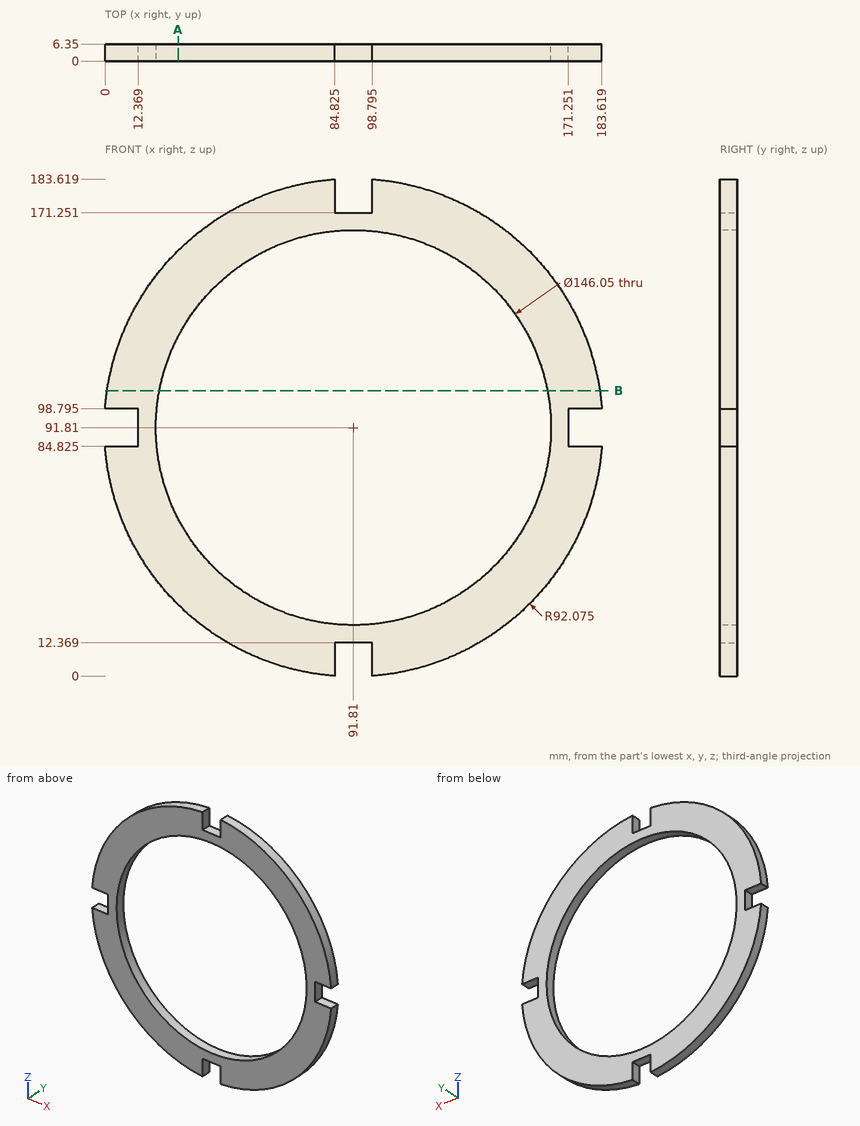
Answer from the drawing. Dimensions are ordinates in mm from the lowest x, y and z of the part. Round coordinates to 2 decimals unless told otherwise and drop trailing zeros. Order: outer loops, then holes, each group sorted by start corner. A loop starts at its lowest first (then second) coordinate and runs counter-clockwise, first axis right, second up. Notation, with made-up numbers: (41, 23.25) -> (90, 23.25) arc R31 ccw to (90, 58.25) -> close; hole circle Ø1 at (33, 70.5). An arc over 180 degrees is marked (long way). Answer as CSV lines item,"result".
Q1. A cutting plane is placed at A-A on x = 27. Determine the outline of the cut face in (y, z).
Computed values:
outline,"(0, 26.41) -> (6.35, 26.41) -> (6.35, 58.16) -> (0, 58.16) -> close; (0, 125.46) -> (6.35, 125.46) -> (6.35, 157.21) -> (0, 157.21) -> close"
Q2. A cutting plane is placed at B-B on z = 105.5. Determine the outline of the cut face in (x, y).
Computed values:
outline,"(0.76, 0) -> (20.08, 0) -> (20.08, 6.35) -> (0.76, 6.35) -> close; (163.54, 0) -> (182.86, 0) -> (182.86, 6.35) -> (163.54, 6.35) -> close"
Q3. Consider line 1 (X direction, y = 4, z = 119.5); line 2 (X direction, y = 1.75, z = 141) (1 decimal); line 3 (Z direction, x = 59, y = 1). Determine where each line is inside the solid, lowest interval first. Write a range as from..to.
Computed values:
line 1,"x = 4..24.24, 159.38..179.62"
line 2,"x = 14..37.8, 145.8..169.6"
line 3,"z = 5.78..26.57, 157.05..177.84"
Q4. Given pin 1 (1 mm diameter, centred on x = 23.5, y = 5.5, fed in from -Z); pin 2 (3 mm diameter, centred on y = 3, z = 175, fed in from -X); pin 3 (1.9 mm diameter, centred on x = 89.5, y = 4, fed in from +Z), each flat-ended and moving along its own axis, determine where each tip first touches the part or whether it passes through.
Computed values:
pin 1,"stops at z = 29.52"
pin 2,"stops at x = 49.33"
pin 3,"stops at z = 171.25"
